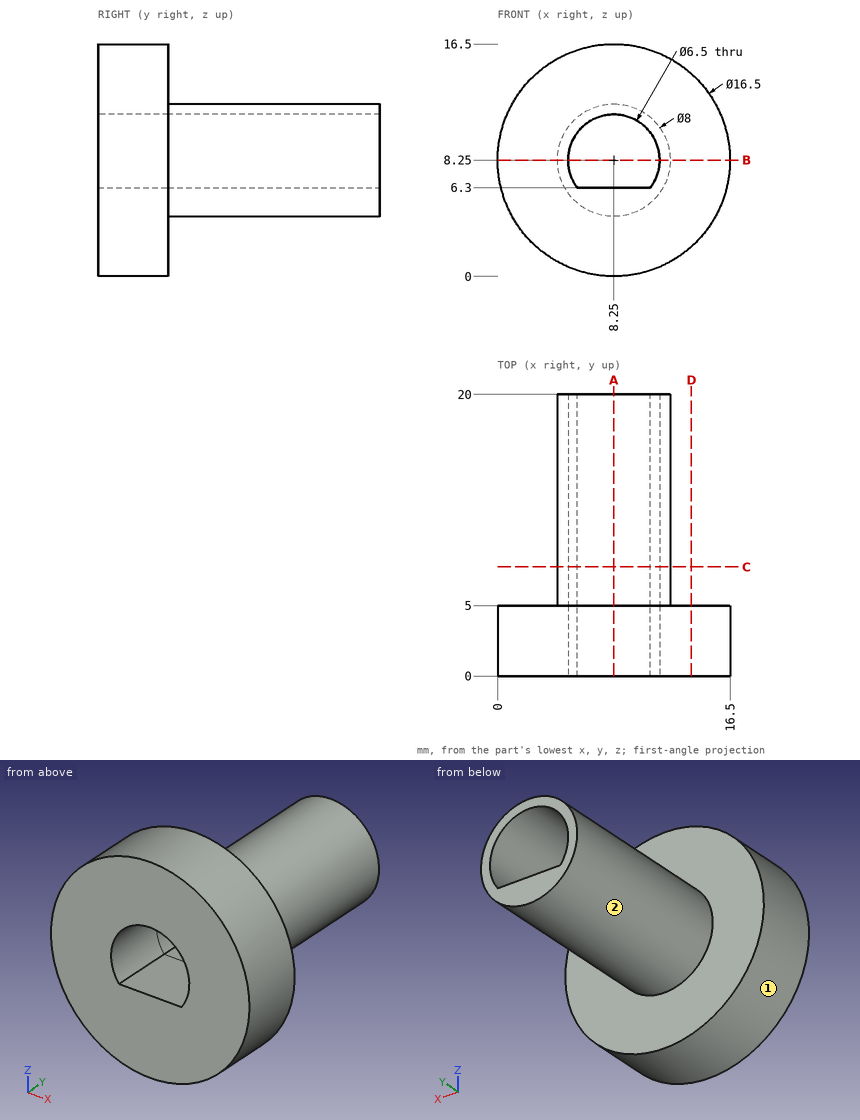
Geometry check sheet. Reference: drawing and pictorial views, mm from the part's lowest x, y, z. A direction names the side the tool comes from. Give positions to 0.01 mm unless a question says otherwise; leave off trailing zeros. Loops run counter-clockwise (first coordinate to the right, second up) from the corner with the lowest first, then second, coordinate; pieces in that order, holes last. Notation, with made-up numbers: (54.5, 70) -> (112.5, 70) arc R36 ccw to (112.5, 107) -> close; hole circle Ø4 at (15, -12.5). An arc over 180 degrees is marked (long way). Answer in a Markdown table with one row per item. Add a question column.
1) Cross-section at C-C on y = 7.75. Record the boundary of the cut face in (x, z).
2) Cross-section at A-A on x = 8.25. Record the boundary of the cut face in (y, z), and give its area (3 significant figures).
3) Gauge pin test, flat ends, axial feed: P1, Ø5, axis at x = 5, y = 9.5, coming from the +Z side; P2, Ø2, axis at y = 15, z = 8, coming from the +X side; P3, Ø1.5, axis at y = 9, z = 14, coming from the -X side. Record the tip position at first contact, or that the pin passes through.
4) Set-up check for the marked faces 1 and 2: record each of +Z, -Z, +X, -X, +Y, -Y from which the full face is reachable in a straight line by a thin tool's end or side.
5) Cross-section at B-B on z = 8.25. Record the boundary of the cut face in (x, y).
6) Material ranges on probe 1 along X at (y, z) = (2.1, 8.25); probe 2 along X at (y, z) = (9.5, 8.25); probe 3 along Y at (x, z) = (15, 4.75), recorded low to high. Write a range as from..to.
7) Cross-section at D-D on x = 13.75. Record the boundary of the cut face in (y, z).
Outcome:
| question | item | result |
|---|---|---|
| 1 | outline | circle Ø8 at (8.25, 8.25); hole (5.65, 6.3) -> (10.85, 6.3) arc R3.25 ccw (long way) to start |
| 2 | outline | (0, 0) -> (5, 0) -> (5, 4.25) -> (20, 4.25) -> (20, 6.3) -> (0, 6.3) -> close; (0, 11.5) -> (20, 11.5) -> (20, 12.25) -> (5, 12.25) -> (5, 16.5) -> (0, 16.5) -> close |
| 2 | area | 98.5 mm^2 |
| 3 | P1 | stops at z = 12.18 |
| 3 | P2 | stops at x = 12.25 |
| 3 | P3 | passes through |
| 4 | face 1 | +Y, -Y |
| 4 | face 2 | +Y |
| 5 | outline | (0, 0) -> (5, 0) -> (5, 20) -> (4.25, 20) -> (4.25, 5) -> (0, 5) -> close; (11.5, 0) -> (16.5, 0) -> (16.5, 5) -> (12.25, 5) -> (12.25, 20) -> (11.5, 20) -> close |
| 6 | probe 1 | x = 0..5, 11.5..16.5 |
| 6 | probe 2 | x = 4.25..5, 11.5..12.25 |
| 6 | probe 3 | y = 0..5 |
| 7 | outline | (0, 2.1) -> (5, 2.1) -> (5, 14.4) -> (0, 14.4) -> close |
